Read the model definition and answer for the solid it produces. Units are mm, in the model's axes. A direction names the side the tool comes from. Give positions to 0.01 mm unless a question says otherwise; leave off trailing zeros. Write each loop counter-clockwise with the first axis right and the second up, starting at its lowest first coordinate (ties: lowest second). Pieces come first, ordered by that corner, then holes. Notation, with made-up numbers: (-34.5, 62.25) - (-1.5, 62.25) arc R17 ccw to (-1.5, 68.25) - close; hole circle Ø11 at (50, 33). An arc over 180 degrees is marked (long way). Answer as CSV lines item,"result".
```python
from build123d import *

# Parameters (mm, degrees)
SKETCH2_W       = 47.752
SKETCH2_H       = 4.7625
LPATTERN1_COUNT = 4
LPATTERN1_PITCH = 3.6068
SKETCH6_W       = 4.7625
SKETCH6_H       = 27.2415
LPATTERN2_COUNT = 4
LPATTERN2_PITCH = 3.6068
SKETCH5_W       = 57.104130169
SKETCH5_H       = 1.6256
SKETCH9_W       = 1.6256
SKETCH9_H       = 27.2415
CHAMFER1_SIZE   = 0.127
FILLET1_R       = 0.127


with BuildPart() as part:
    # Sketch2 → Revolve1 (revolve)
    with BuildSketch(Plane(origin=(0, 0, 0), x_dir=(0, 0, -1), z_dir=(1, 0, 0)), mode=Mode.PRIVATE) as revolve1_sk:
        with Locations((0, 2.38125)):
            Rectangle(SKETCH2_W, SKETCH2_H)
    revolve(revolve1_sk.sketch.rotate(Axis((0, 0, 23.876), (0, 0, -1)), 90), axis=Axis((0, 0, 23.876), (0, 0, -1)))

    # Sketch3 → Cut-Revolve1 (revolve, cut)
    with BuildSketch(Plane(origin=(0, 0, 0), x_dir=(0, 0, -1), z_dir=(1, 0, 0)), mode=Mode.PRIVATE) as cut_revolve1_sk:
        Polygon((-23.876, 4.7625), (-23.876, 2.38125), (-9.4488, 2.38125), (-5.842, 2.921), (-5.842, 4.7625), align=None)
    cut_revolve1 = revolve(cut_revolve1_sk.sketch.rotate(Axis((0, 0, 23.876), (0, 0, -1)), 90), axis=Axis((0, 0, 23.876), (0, 0, -1)), mode=Mode.SUBTRACT)

    # Sketch4 → Revolve2 (revolve)
    with BuildSketch(Plane(origin=(0, 0, 0), x_dir=(0, 0, -1), z_dir=(1, 0, 0))):
        Polygon((-20.2692, 2.921), (-20.3962, 2.921), (-23.876, 2.38125), (-20.2692, 2.38125), align=None)
    revolve2 = revolve(axis=Axis((0, 0, 5.842), (0, 0, 1)))

    # LPattern1: Revolve2 ×4
    with Locations(*[(0, 0, -i * LPATTERN1_PITCH) for i in range(1, LPATTERN1_COUNT)]):
        add(revolve2)

    # Mirror1: Cut-Revolve1, Revolve2 across plane
    add(cut_revolve1.mirror(Plane.XY), mode=Mode.SUBTRACT)
    add(revolve2.mirror(Plane.XY))

    # Mirror1 copy 1 sketch → Mirror1 copy 1 (revolve)
    with BuildSketch(Plane(origin=(0, 0, 3.6068), x_dir=(0, 0, 1), z_dir=(1, 0, 0))):
        Polygon((-20.2692, -2.921), (-20.3962, -2.921), (-23.876, -2.38125), (-20.2692, -2.38125), align=None)
    revolve(axis=Axis((0, 0, -2.2352), (0, 0, 1)))

    # Mirror1 copy 2 sketch → Mirror1 copy 2 (revolve)
    with BuildSketch(Plane(origin=(0, 0, 7.2136), x_dir=(0, 0, 1), z_dir=(1, 0, 0))):
        Polygon((-20.2692, -2.921), (-20.3962, -2.921), (-23.876, -2.38125), (-20.2692, -2.38125), align=None)
    revolve(axis=Axis((0, 0, 1.3716), (0, 0, 1)))

    # Mirror1 copy 3 sketch → Mirror1 copy 3 (revolve)
    with BuildSketch(Plane(origin=(0, 0, 10.8204), x_dir=(0, 0, 1), z_dir=(1, 0, 0))):
        Polygon((-20.2692, -2.921), (-20.3962, -2.921), (-23.876, -2.38125), (-20.2692, -2.38125), align=None)
    revolve(axis=Axis((0, 0, 4.9784), (0, 0, 1)))

    # Sketch6 → Revolve3 (revolve)
    with BuildSketch(Plane(origin=(0, 0, 0), x_dir=(0, 0, -1), z_dir=(1, 0, 0)), mode=Mode.PRIVATE) as revolve3_sk:
        with Locations((-2.38125, 13.62075)):
            Rectangle(SKETCH6_W, SKETCH6_H)
    revolve(revolve3_sk.sketch.rotate(Axis((0, 0, 0), (0, 1, 0)), 180), axis=Axis((0, 0, 0), (0, 1, 0)))

    # Sketch7 → Cut-Revolve3 (revolve, cut)
    with BuildSketch(Plane(origin=(0, 0, 0), x_dir=(0, 0, -1), z_dir=(1, 0, 0)), mode=Mode.PRIVATE) as cut_revolve3_sk:
        Polygon((-2.921, 9.2075), (-2.38125, 12.8143), (-2.38125, 27.2415), (-4.7625, 27.2415), (-4.7625, 9.2075), align=None)
    revolve(cut_revolve3_sk.sketch.rotate(Axis((0, 0, 0), (0, 1, 0)), 180), axis=Axis((0, 0, 0), (0, 1, 0)), mode=Mode.SUBTRACT)

    # Sketch8 → Revolve4 (revolve)
    with BuildSketch(Plane(origin=(0, 0, 0), x_dir=(0, 0, -1), z_dir=(1, 0, 0)), mode=Mode.PRIVATE) as revolve4_sk:
        Polygon((-2.38125, 27.2415), (-2.921, 23.7617), (-2.921, 23.6347), (-2.38125, 23.6347), align=None)
    revolve4 = revolve(revolve4_sk.sketch.rotate(Axis((0, 27.2415, 0), (0, -1, 0)), 180), axis=Axis((0, 27.2415, 0), (0, -1, 0)))

    # LPattern2: Revolve4 ×4
    with Locations(*[(0, -i * LPATTERN2_PITCH, 0) for i in range(1, LPATTERN2_COUNT)]):
        add(revolve4)

    # Sketch5 → Cut-Revolve2 (revolve, cut)
    with BuildSketch(Plane(origin=(0, 0, 0), x_dir=(0, 0, -1), z_dir=(1, 0, 0))):
        with Locations((4.676065085, 0.8128)):
            Rectangle(SKETCH5_W, SKETCH5_H)
    revolve(axis=Axis((0, 0, 23.876), (0, 0, -1)), mode=Mode.SUBTRACT)

    # Sketch9 → Cut-Revolve4 (revolve, cut)
    with BuildSketch(Plane(origin=(0, 0, 0), x_dir=(0, 0, -1), z_dir=(1, 0, 0))):
        with Locations((-0.8128, 13.62075)):
            Rectangle(SKETCH9_W, SKETCH9_H)
    revolve(axis=Axis((0, 27.2415, 0), (0, -1, 0)), mode=Mode.SUBTRACT)

    # Chamfer1
    chamfer1_edges = [part.edges().sort_by_distance(p)[0] for p in [
        (-4.7625, 0, -5.842),
        (0, 9.2075, 4.7625),
        (-4.7625, 0, 5.842),
    ]]
    chamfer(chamfer1_edges, length=CHAMFER1_SIZE)

    # Fillet1
    fillet1_edges = [part.edges().sort_by_distance(p)[0] for p in [
        (0, -2.38125, 23.876),
        (0, -2.38125, -23.876),
        (0, 27.2415, 2.38125),
    ]]
    fillet(fillet1_edges, radius=FILLET1_R)


solid = part.part
```
(1) A cutting plane is placed at A-A (y = 8). Write down the section's boundary in (x, z) (1 decimal).
Worked out:
outline,"circle Ø9.5 at (0, 0); hole circle Ø3.3 at (0, 0)"
(2) For faces 1 (the conical face through (-2.576, -0.338, -22.481)), 2 (the cylindrical face through (-1.431, 5.613, -4.543)), 3 (the conical face through (1.2, 2.3, 8.02)), determine the directions among +Z, -Z, +X, -X, +Y, -Y from which every point of the face is accessible in a straight line to the end or side of a thin tool.
Worked out:
face 1,"-Z"
face 2,"+Y"
face 3,"none"
(3) The mould has two halves that part along Z. Classify faces 4 (the flat face through (1, 27.242, -1.5)), 5 (the flat face through (-1, 1.5, -23.876)), 6 (the cylindrical face through (-1.61, 13.81, -0.21)): +Z half, -Z half, draft (parallel to the pull), parting line (faces both ways), or undercut.
Worked out:
face 4,"draft"
face 5,"-Z half"
face 6,"undercut"
(4) Each of these flat-tipped pins is pushed along its axis until it touches: P1, Ø3, axis at x = -1.5, y = 0.5, coming from the -Z side; P2, Ø1.5, axis at x = -1.5, z = -13.5, coming from the +Y side; P3, Ø1.5, axis at y = -1, z = -3.5, coming from the -X side; P4, Ø3, axis at x = 1.5, y = 6, coming from the -Z side. Where does it stop, or does it pass through?
Worked out:
P1,"stops at z = -23.88"
P2,"stops at y = 2.8"
P3,"stops at x = -4.76"
P4,"stops at z = -5.79"
(5) Find the intervals of material crossed by L1, parallel to X at y = 7.5, z = 0; L2, parallel to Z at x = -3, y = 1; L3, parallel to X at y = 0, z = 12.5, in increasing order.
Worked out:
L1,"x = -4.76 to -1.63, 1.63 to 4.76"
L2,"z = -5.84 to 5.84"
L3,"x = -2.47 to -1.63, 1.63 to 2.47"
(6) A cutting plane is placed at C-C (z = 19). Write down the section's boundary in (x, y), and give its area (3 significant figures).
Worked out:
outline,"circle Ø5.16 at (0, 0); hole circle Ø3.25 at (0, 0)"
area,"12.6 mm^2"
(7) A cutting plane is placed at B-B (x = 0). Count the separate pieces of the cut face and the enclosed holes in it, and give its area (3 significant figures).
Worked out:
separate pieces,"3"
enclosed holes,"0"
area,"203 mm^2"
